Part model, mm, in its own coordinate system. A direction names the side the tool comes from. Give positions to 0.01 mm unless a question says otherwise; leave off trailing zeros. Write each loop counter-clockwise with the first axis right and the second up, starting at its lowest first coordinate (ties: lowest second). Pieces come first, ordered by that corner, then holes. Notation, with made-up numbers: M 43,87.25 L 76,87.25 A13 ccw 76,106.25 Z; hole C 26,48.5 d8. An arc over 180 degrees is marked long. Use a Markdown table: item, result. Add a question column.
from build123d import *

# Parameters (mm, degrees)
F1_DEPTH = 3
F2_R     = 2.5
F3_DEPTH = 2
F4_R     = 1.25
F5_DEPTH = 4
F6_R     = 3
F6_R_2   = 2.5
F7_DEPTH = 2


with BuildPart() as f1:
    # F0 (on Front) → F1 (new body)
    with BuildSketch(Plane.XZ):
        Polygon((-16, 0), (0, 0), (0, 24), (-8, 24), align=None)
    extrude(amount=F1_DEPTH)

    # F2 (on face) → F3 (join)
    with BuildSketch(Plane(origin=(0, 0, 0), x_dir=(-1, 0, 0), z_dir=(0, 1, 0))):
        with Locations((4, 20)):
            Circle(F2_R)
        with Locations((4, 12)):
            Circle(F2_R)
        with Locations((4, 4)):
            Circle(F2_R)
    extrude(amount=F3_DEPTH)

    # F4 (on face) → F5 (cut)
    with BuildSketch(Plane.XZ.offset(3)):
        with Locations((-4, 20)):
            Circle(F4_R)
        with Locations((-4, 12)):
            Circle(F4_R)
        with Locations((-4, 4)):
            Circle(F4_R)
    extrude(amount=-F5_DEPTH, mode=Mode.SUBTRACT)

    # F6 (on face) → F7 (cut)
    with BuildSketch(Plane.XZ.offset(3)):
        with BuildLine():
            Line((-13.9188611699, 1.5), (-1.5, 1.5))
            Line((-1.5, 1.5), (-1.5, 22.5))
            Line((-1.5, 22.5), (-6.9188611699, 22.5))
            Line((-6.9188611699, 22.5), (-8.0859382195, 18.9987688511))
            ThreePointArc((-8.0859382195, 18.9987688511), (-5.1539501058, 15.0513167019), (-9.8680118863, 13.6525478508))
            Line((-9.8680118863, 13.6525478508), (-10.6400973399, 14.0977761451))
            ThreePointArc((-10.6400973399, 14.0977761451), (-10.9160755398, 14.2527999833), (-11.209430585, 14.3717082451))
            Line((-11.209430585, 14.3717082451), (-12.790569415, 9.6282917549))
            Line((-12.790569415, 9.6282917549), (-11.367544468, 9.1539501058))
            Line((-11.367544468, 9.1539501058), (-12.2565955429, 6.486796881))
            Line((-12.2565955429, 6.486796881), (-13.67962049, 6.96113853))
            Line((-13.67962049, 6.96113853), (-15.12037951, 2.63886147))
            Line((-15.12037951, 2.63886147), (-13.6973545629, 2.1645198209))
            Line((-13.6973545629, 2.1645198209), (-13.9188611699, 1.5))
        make_face()
        with Locations((-8, 8)):
            Circle(F6_R, mode=Mode.SUBTRACT)
        with BuildLine():
            Line((-8.2565955429, 18.486796881), (-9.6973545629, 14.1645198209))
            ThreePointArc((-9.6973545629, 14.1645198209), (-5.6282917549, 15.209430585), (-8.2565955429, 18.486796881))
        make_face()
        with Locations((-8, 8)):
            Circle(F6_R_2)
    extrude(amount=-F7_DEPTH, mode=Mode.SUBTRACT)


solid = f1.part
1. Tool access for faces 1 (the flat face through (-1.5, -2, 12)), 2 (the flat face through (-13, -3, 8)): list every direction of +Z, -Z, +X, -X, +Y, -Y with a clear straight run to the whole face (end or side of a thin tool).
2. Flat gauge pins, fed straight in: pin 1 (1 mm diameter, centred on x = -5, z = 7, fed in from +Y); pin 2 (0.8 mm diameter, centred on x = -3.5, z = 4.5, fed in from -Y); pin 3 (2 mm diameter, centred on x = -4.5, z = 20, fed in from -Y). Where does each tip first touch, or does it go through?
3. Cut at C-C (z = 16). Write the cut outline in (x, y).
4. Cut at A-A (y = -1.45). Write the cut outline in (x, z), then the cut area to 3 significant figures.
5. Drill centre lines: probe 1 along Z at (x, y) = (-4, 0.55); probe 2 along X at (y, z) = (-2, 16); probe 3 along Y at (x, z) = (-2.5, 2.25). Where is each one in solid material? Low to high. Write a range as [from, to].
6. Cut at B-B (y = 0.4). Write the cut outline in (x, z), then the cut area to 3 significant figures.
7. Mould opens along X. For faces 3 (the flat face through (-11.944, -0.812, 12.168)), 4 (the cylindrical face through (-5.13, -2.01, 15.13)), 5 (the flat face through (-6, 0, 10)) say: released by +X, released by -X, zero draft, split by the parting line, or undercut.
A:
| question | item | result |
|---|---|---|
| 1 | face 1 | -Y |
| 1 | face 2 | +Z, -Z, +X, -X, -Y |
| 2 | pin 1 | stops at y = 0 |
| 2 | pin 2 | stops at y = 1 |
| 2 | pin 3 | stops at y = -1 |
| 3 | outline | M -10.67,-3 L -9.09,-3 L -9.09,-1 L -5.5,-1 L -5.5,-3 L -5,-3 L -5,-1 L -1.5,-1 L -1.5,-3 L 0,-3 L 0,0 L -10.67,0 Z |
| 4 | outline | M -16,0 L 0,0 L 0,24 L -8,24 L -11.21,14.37 A2.5 cw -10.64,14.1 L -9.87,13.65 A3 ccw long -8.09,19 L -6.92,22.5 L -1.5,22.5 L -1.5,1.5 L -13.92,1.5 L -13.7,2.16 L -15.12,2.64 Z; M -13.68,6.96 L -12.26,6.49 L -11.37,9.15 L -12.79,9.63 Z; C -8,8 d6; hole C -8,8 d5; hole M -9.7,14.16 A2.5 ccw long -8.26,18.49 Z |
| 4 | area | 101 mm² |
| 5 | probe 1 | z = [1.5, 2.75], [5.25, 6.5], [9.5, 10.75], [13.25, 14.5], [17.5, 18.75], [21.25, 22.5] |
| 5 | probe 2 | x = [-10.67, -9.09], [-5.5, -5], [-1.5, 0] |
| 5 | probe 3 | y = [-1, 2] |
| 6 | outline | C -4,4 d5; C -4,12 d5; C -4,20 d5; hole C -4,4 d2.5; hole C -4,12 d2.5; hole C -4,20 d2.5 |
| 6 | area | 44.2 mm² |
| 7 | face 3 | released by -X |
| 7 | face 4 | undercut |
| 7 | face 5 | zero draft |
